Here's how the part is built. I have some questions about the finished solid (model axes, mm). Face numbers are marked on the shaded views. A direction names the side the tool comes from. Coordinates: 2 decimals unless noted, no trailing zeros. Order: outer loops, then holes, each group sorted by start corner. A loop starts at its lowest first (then second) coordinate and runs counter-clockwise, first axis right, second up. Notation, with made-up numbers: (39.5, 6) - (44.5, 6) arc R20 cw to (44.5, 35) - close; hole circle Ø5 at (44.25, 33). An arc over 180 degrees is marked (long way). Answer in a Markdown table with one row per item. Add a question column.
Item 1: On a 3-axis mill with a long thin cutter (end or side, diameter ignored), from which of +Z, -Z, +X, -X, +Y, -Y can I reach the whole of each face in a straight line? I mean the marked faces 5 and 6. Say none if no direction works.
Item 2: Will these pins go through, and if not, where does the flat tip stop? pin 1 Ø3.5 at (x, y) = (0, 7) entering from -Z; pin 2 Ø6.5 at (x, z) = (-19, 0) entering from +Y; pin 3 Ø4 at (x, y) = (7, 6.5) entering from +Z.
Item 3: I want a section at A-A (x = 0). Please give me the cut outline in (y, z), plus the area to 3 significant figures.
Item 4: I want a section at B-B (z = 0). Please give me the cut outline in (x, y), plus the area to 3 significant figures.
Item 5: Thinking about a two-plate mould opening in X: for the marked faces 1, 2, 3 and 4, which applies, +X half, -X half, draft (parallel to the pull), parting line (faces both ways), or undercut?
Item 6: If I drill on line 1 along Z through (x, y) = (12.5, 0.5); line 2 along Y through (x, z) = (-8, 20); line 3 along X through (y, z) = (6.5, 1.5), over which ranges is the centre line in solid material (lowest first)? Write a range as from..to.
Item 7: I want a section at D-D (y = 7). Please give me the cut outline in (x, z), plus the area to 3 significant figures.
Item 8: I want a section at C-C (x = -19). Please give me the cut outline in (y, z), plus the area to 3 significant figures.
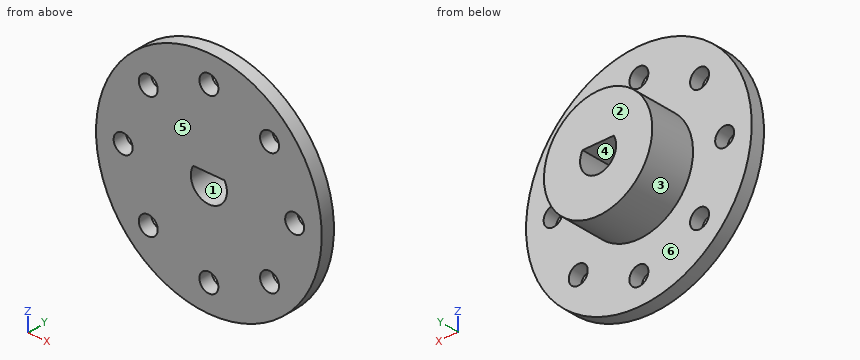
```python
from build123d import *

# Parameters (mm, degrees)
SKETCH_1_R          = 25
SKETCH_1_R_2        = 2.1
EXTRUDE_1_DEPTH     = 3
SKETCH_2_R          = 12
EXTRUDE_2_DEPTH     = 10
CUT_EXTRUDE_START   = -20
CUT_EXTRUDE_1_DEPTH = 20


with BuildPart() as part:
    # 草图1 → 凸台-拉伸1 (new body)
    with BuildSketch(Plane(origin=(0, 0, 0), x_dir=(1, 0, 0), z_dir=(0, 1, 0))):
        with Locations(Location((0, 0, 0), (0, 0, 270))):
            Circle(SKETCH_1_R)
        with Locations(Location((0, 19, 0), (0, 0, 270))):
            Circle(SKETCH_1_R_2, mode=Mode.SUBTRACT)
        with Locations(Location((13.435028843, 13.435028843, 0), (0, 0, 270))):
            Circle(SKETCH_1_R_2, mode=Mode.SUBTRACT)
        with Locations(Location((19, 0, 0), (0, 0, 270))):
            Circle(SKETCH_1_R_2, mode=Mode.SUBTRACT)
        with Locations(Location((13.435028843, -13.435028843, 0), (0, 0, 270))):
            Circle(SKETCH_1_R_2, mode=Mode.SUBTRACT)
        with Locations(Location((0, -19, 0), (0, 0, 270))):
            Circle(SKETCH_1_R_2, mode=Mode.SUBTRACT)
        with Locations(Location((-13.435028843, -13.435028843, 0), (0, 0, 270))):
            Circle(SKETCH_1_R_2, mode=Mode.SUBTRACT)
        with Locations(Location((-19, 0, 0), (0, 0, 270))):
            Circle(SKETCH_1_R_2, mode=Mode.SUBTRACT)
        with Locations(Location((-13.435028843, 13.435028843, 0), (0, 0, 270))):
            Circle(SKETCH_1_R_2, mode=Mode.SUBTRACT)
    extrude(amount=EXTRUDE_1_DEPTH)

    # 草图2 → 凸台-拉伸2 (add)
    with BuildSketch(Plane(origin=(0, 3, 0), x_dir=(1, 0, 0), z_dir=(0, 1, 0))):
        with Locations(Location((0, 0, 0), (0, 0, 270))):
            Circle(SKETCH_2_R)
        with BuildLine():
            Line((-3.464101615, -2), (3.464101615, -2))
            ThreePointArc((3.464101615, -2), (0, 4), (-3.464101615, -2))
        make_face(mode=Mode.SUBTRACT)
    extrude(amount=EXTRUDE_2_DEPTH)

    # 草图3 → 切除-拉伸1 (cut)
    with BuildSketch(Plane(origin=(0, 13, 0), x_dir=(1, 0, 0), z_dir=(0, 1, 0)).offset(CUT_EXTRUDE_START)):
        with BuildLine():
            Line((-3.464101615, -2), (3.464101615, -2))
            ThreePointArc((3.464101615, -2), (0, 4), (-3.464101615, -2))
        make_face()
    extrude(amount=CUT_EXTRUDE_1_DEPTH, mode=Mode.SUBTRACT)


solid = part.part
```
Values follow:
| question | item | result |
|---|---|---|
| 1 | face 5 | +Z, -Z, +X, -X, -Y |
| 1 | face 6 | +Y |
| 2 | pin 1 | stops at z = -12 |
| 2 | pin 2 | stops at y = 3 |
| 2 | pin 3 | stops at z = 10.91 |
| 3 | outline | (0, -25) - (3, -25) - (3, -21.1) - (0, -21.1) - close; (0, -16.9) - (3, -16.9) - (3, -12) - (13, -12) - (13, -4) - (0, -4) - close; (0, 2) - (13, 2) - (13, 12) - (3, 12) - (3, 16.9) - (0, 16.9) - close; (0, 21.1) - (3, 21.1) - (3, 25) - (0, 25) - close |
| 3 | area | 287 mm^2 |
| 4 | outline | (-25, 0) - (-21.1, 0) - (-21.1, 3) - (-25, 3) - close; (-16.9, 0) - (-4, 0) - (-4, 13) - (-12, 13) - (-12, 3) - (-16.9, 3) - close; (4, 0) - (16.9, 0) - (16.9, 3) - (12, 3) - (12, 13) - (4, 13) - close; (21.1, 0) - (25, 0) - (25, 3) - (21.1, 3) - close |
| 4 | area | 261 mm^2 |
| 5 | face 1 | undercut |
| 5 | face 2 | draft |
| 5 | face 3 | parting line |
| 5 | face 4 | undercut |
| 6 | line 1 | z = -21.65..-15.32, -11.55..11.55, 15.32..21.65 |
| 6 | line 2 | y = 0..3 |
| 6 | line 3 | x = -11.91..-3.71, 3.71..11.91 |
| 7 | outline | circle Ø24 at (0, 0); hole (-3.46, 2) arc R4 ccw (long way) to (3.46, 2) - close |
| 7 | area | 412 mm^2 |
| 8 | outline | (0, -16.25) - (3, -16.25) - (3, -2.1) - (0, -2.1) - close; (0, 2.1) - (3, 2.1) - (3, 16.25) - (0, 16.25) - close |
| 8 | area | 84.9 mm^2 |
